from build123d import *

# Parameters (mm, degrees)
SKETCH_1_W           = 7.8
SKETCH_1_H           = 83.4
EXTRUDE_1_DEPTH      = 105
CUT_EXTRUDE_1_DEPTH  = 135.318278726
SKETCH_3_R           = 6
CUT_EXTRUDE_2_DEPTH  = 135.318278726
SKETCH_4_R           = 13.6
CUT_EXTRUDE_3_DEPTH  = 4
SKETCH_5_R           = 1.25
CUT_EXTRUDE_4_DEPTH  = 4
EXTRUDE_2_DEPTH      = 7.2
SKETCH_7_W           = 6
SKETCH_7_H           = 30
CUT_EXTRUDE_5_DEPTH  = 7.2
CUT_EXTRUDE_6_DEPTH  = 135.92798079
SKETCH_9_R           = 1.65
CUT_EXTRUDE_7_DEPTH  = 15
FILLET_1_R           = 5
CUT_EXTRUDE_8_DEPTH  = 135.92798079
CUT_EXTRUDE_10_DEPTH = 135.92798079
SKETCH_14_R          = 1.6
CUT_EXTRUDE_11_DEPTH = 135.92798079
SKETCH_15_R          = 3
CUT_EXTRUDE_12_DEPTH = 2


with BuildPart() as part:
    # 草图1 → 凸台-拉伸1 (new body)
    with BuildSketch(Plane(origin=(0, 0, 0), x_dir=(1, 0, 0), z_dir=(0, 1, 0))):
        with Locations((3.9, -41.7)):
            Rectangle(SKETCH_1_W, SKETCH_1_H)
    extrude(amount=EXTRUDE_1_DEPTH)

    # 草图2 → 切除-拉伸1 (cut, through all)
    with BuildSketch(Plane.ZY):
        with BuildLine():
            Line((0, 64.3), (0, 105))
            Line((0, 105), (32.622555426, 105))
            ThreePointArc((32.622555426, 105), (9.162180169, 90.380266115), (0, 64.3))
        make_face()
        with BuildLine():
            Line((83.4, 105), (83.4, 64.3))
            ThreePointArc((83.4, 64.3), (74.237819831, 90.380266115), (50.777444574, 105))
            Line((50.777444574, 105), (83.4, 105))
        make_face()
    extrude(amount=-CUT_EXTRUDE_1_DEPTH, mode=Mode.SUBTRACT)

    # 草图3 → 切除-拉伸2 (cut, through all)
    with BuildSketch(Plane.ZY):
        with Locations((41.7, 64.3)):
            Circle(SKETCH_3_R)
    extrude(amount=-CUT_EXTRUDE_2_DEPTH, mode=Mode.SUBTRACT)

    # 草图4 → 切除-拉伸3 (cut)
    with BuildSketch(Plane.ZY):
        with Locations((41.7, 64.3)):
            Circle(SKETCH_4_R)
    extrude(amount=-CUT_EXTRUDE_3_DEPTH, mode=Mode.SUBTRACT)

    # 草图5 → 切除-拉伸4 (cut)
    with BuildSketch(Plane.ZY.offset(-4)):
        with Locations((32.2, 64.3)):
            Circle(SKETCH_5_R)
        with Locations((51.2, 64.3)):
            Circle(SKETCH_5_R)
    extrude(amount=-CUT_EXTRUDE_4_DEPTH, mode=Mode.SUBTRACT)

    # 草图6 → 凸台-拉伸2 (add)
    with BuildSketch(Plane(origin=(7.8, 0, 0), x_dir=(0, 0, -1), z_dir=(1, 0, 0))):
        with BuildLine():
            ThreePointArc((-14.146415841, 30), (-26.974511893, 22.286540784), (-41.7, 19.6))
            Line((-41.7, 19.6), (-41.7, 0))
            Line((-41.7, 0), (0, 0))
            Line((0, 0), (0, 30))
            Line((0, 30), (-14.146415841, 30))
        make_face()
        with BuildLine():
            Line((-41.7, 0), (-41.7, 19.6))
            ThreePointArc((-41.7, 19.6), (-56.425488107, 22.286540784), (-69.253584159, 30))
            Line((-69.253584159, 30), (-83.4, 30))
            Line((-83.4, 30), (-83.4, 0))
            Line((-83.4, 0), (-41.7, 0))
        make_face()
    extrude(amount=EXTRUDE_2_DEPTH)

    # 草图7 → 切除-拉伸5 (cut)
    with BuildSketch(Plane(origin=(15, 0, 0), x_dir=(0, 0, -1), z_dir=(1, 0, 0))):
        with Locations((-80.4, 15)):
            Rectangle(SKETCH_7_W, SKETCH_7_H)
    extrude(amount=-CUT_EXTRUDE_5_DEPTH, mode=Mode.SUBTRACT)

    # 草图8 → 切除-拉伸6 (cut, through all)
    with BuildSketch(Plane.ZY):
        with BuildLine():
            Line((31.7, 17), (51.7, 17))
            ThreePointArc((51.7, 17), (55.235533906, 15.535533906), (56.7, 12))
            Line((56.7, 12), (56.7, 0))
            Line((56.7, 0), (26.7, 0))
            Line((26.7, 0), (26.7, 12))
            ThreePointArc((26.7, 12), (28.164466094, 15.535533906), (31.7, 17))
        make_face()
    extrude(amount=-CUT_EXTRUDE_6_DEPTH, mode=Mode.SUBTRACT)

    # 草图9 → 切除-拉伸7 (cut)
    with BuildSketch(Plane.XZ):
        with Locations(Location((7.5, 73.4, 0), (0, 0, 270))):
            Circle(SKETCH_9_R)
        with Locations(Location((7.5, 62.7, 0), (0, 0, 270))):
            Circle(SKETCH_9_R)
        with Locations(Location((7.5, 20.7, 0), (0, 0, 270))):
            Circle(SKETCH_9_R)
        with Locations(Location((7.5, 6, 0), (0, 0, 270))):
            Circle(SKETCH_9_R)
    extrude(amount=-CUT_EXTRUDE_7_DEPTH, mode=Mode.SUBTRACT)


with BuildPart() as body_2:
    # 镜向2: mirrored copy
    add(part.part.mirror(Plane(origin=(0, 0, 0), x_dir=(0, 0, 1), z_dir=(1, 0, 0))))

    # 圆角1
    fillet_1_edges = [body_2.edges().sort_by_distance(p)[0] for p in [
        (-11.4, 30, 14.146415841),
        (-11.4, 30, 69.253584159),
    ]]
    fillet(fillet_1_edges, radius=FILLET_1_R)

    # 草图10 → 切除-拉伸8 (cut, through all)
    with BuildSketch(Plane(origin=(0, 0, 0), x_dir=(0, 0, -1), z_dir=(1, 0, 0))):
        with BuildLine():
            ThreePointArc((-37.240706086, 94.065786869), (-59.594392776, 88.500786708), (-71.465786869, 68.759293914))
            ThreePointArc((-71.465786869, 68.759293914), (-68.859293916, 65.234213137), (-65.334213139, 67.840706089))
            ThreePointArc((-65.334213139, 67.840706089), (-55.908255092, 83.515569664), (-38.159293911, 87.934213139))
            ThreePointArc((-38.159293911, 87.934213139), (-34.634213133, 90.540706091), (-37.240706086, 94.065786869))
        make_face()
    extrude(amount=-CUT_EXTRUDE_8_DEPTH, mode=Mode.SUBTRACT)

    # 草图13 → 切除-拉伸10 (cut, through all)
    with BuildSketch(Plane(origin=(0, 0, 0), x_dir=(0, 0, -1), z_dir=(1, 0, 0))):
        with BuildLine():
            ThreePointArc((-56.294598294, 36.728714307), (-54.592965975, 31.672402134), (-51.772187936, 27.144151191))
            ThreePointArc((-51.772187936, 27.144151191), (-44.745463477, 26.353491098), (-43.954803385, 33.380215557))
            ThreePointArc((-43.954803385, 33.380215557), (-45.549156189, 35.939661742), (-46.51094837, 38.797577319))
            ThreePointArc((-46.51094837, 38.797577319), (-52.437204837, 42.654970775), (-56.294598294, 36.728714307))
        make_face()
    extrude(amount=-CUT_EXTRUDE_10_DEPTH, mode=Mode.SUBTRACT)

    # 草图14 → 切除-拉伸11 (cut, through all)
    with BuildSketch(Plane(origin=(0, 0, 0), x_dir=(0, 0, -1), z_dir=(1, 0, 0))):
        with Locations((-79.9, 7)):
            Circle(SKETCH_14_R)
        with Locations((-79.9, 22)):
            Circle(SKETCH_14_R)
    extrude(amount=-CUT_EXTRUDE_11_DEPTH, mode=Mode.SUBTRACT)

    # 草图15 → 切除-拉伸12 (cut)
    with BuildSketch(Plane(origin=(0, 0, 0), x_dir=(0, 0, -1), z_dir=(1, 0, 0))):
        with Locations((-79.9, 22)):
            Circle(SKETCH_15_R)
        with Locations((-79.9, 7)):
            Circle(SKETCH_15_R)
    extrude(amount=-CUT_EXTRUDE_12_DEPTH, mode=Mode.SUBTRACT)


solid = body_2.part
Check sheet for the modelled part. Datum: model origin and axes. Units: mm. A direction names the side the tool comes from. Give positions to 0.01 mm unless a question says otherwise; leave off trailing zeros. Loops run counter-clockwise (first coordinate to the right, second up) from the corner with the lowest first, then second, coordinate; pieces in that order, holes last. Notation, with made-up numbers: M -1.75,69.5 L 36.25,69.5 A8 ccw 36.25,81.5 Z; hole C 27,46.25 d2. An arc over 180 degrees is marked long. Use a Markdown table: item, result. Add a question column.
Q1. Sectioned sample at D-D, the plane z = 79.9. Record the cut outline in (x, y), then the cut area to 3 significant figures.
Q2. Go/stop test with flat-tipped pins: pin 1 (8 mm diameter, centred on x = -5, z = 67.5, fed in from +Y); pin 2 (3.5 mm diameter, centred on y = 7, z = 79.9, fed in from -X); pin 3 (4 mm diameter, centred on x = -7.5, z = 20.7, fed in from -Y); pin 4 (3 mm diameter, centred on y = 8, z = 80.5, fed in from +X). Record where each tip stops, or that it passes through.
Q3. Sectioned sample at C-C, the plane z = 62.7. Record the cut outline in (x, y).
Q4. Sectioned sample at B-B, the plane y = 91. Record the cut outline in (x, z).
Q5. Scan lines: line 1 along Z through (x, y) = (-7.5, 8.75); line 2 along Y through (x, z) = (-4.5, 79.9); line 3 along X through (y, z) = (10.25, 6). Record each from-to range of solid material in increasing order. Write a range as [from, to].
Q6. Tool access check on faces 1 (the cylindrical face through (-3.845, 31.74, 54.625)), 2 (the cylindrical face through (-11.45, 29.705, 69.389)), 3 (the cylindrical face through (-7.57, 7.4, 7.65)), 4 (the flat face through (-2, 5.7, 78.6)), 5 (the flat face through (-7, 6, 26.7)). Record the directions out of +Z, -Z, +X, -X, +Y, -Y that give a thin tool (end or side, any length) a straight path to the whole face; none if there is none.
Q7. Sectioned sample at A-A, the plane x = -12.25. Record the cut outline in (y, z).
Q8. Mould release check, pull along Y, two halves, no side actions. Record for faces 6 (the flat face through (-2, 20.7, 78.6)), 7 (the flat face through (-4, 32, 83.4)), 8 (the flat face through (-8, 15, 21)): pulls with the +Y half, pulls with the -Y half, needs draft (parallel to the pull), parting line crosses it, or undercut.
Verdict:
| question | item | result |
|---|---|---|
| 1 | outline | M -7.8,0 L 0,0 L 0,4 L -2,4 L -2,5.4 L -7.8,5.4 Z; M -7.8,8.6 L -2,8.6 L -2,10 L 0,10 L 0,19 L -2,19 L -2,20.4 L -7.8,20.4 Z; M -7.8,23.6 L -2,23.6 L -2,25 L 0,25 L 0,81.02 L -7.8,81.02 Z |
| 1 | area | 571 mm^2 |
| 2 | pin 1 | y = 99.85 |
| 2 | pin 2 | x = -7.8 |
| 2 | pin 3 | y = 0 |
| 2 | pin 4 | x = -2 |
| 3 | outline | M -15,0 L -9.15,0 L -9.15,15 L -5.85,15 L -5.85,0 L 0,0 L 0,75.71 L -7.8,75.71 L -7.8,25.27 L -15,25.27 Z; M -7.8,85.86 L 0,85.86 L 0,100.33 L -7.8,100.33 Z |
| 4 | outline | M -7.8,9.67 L 0,9.67 L 0,34.6 L -7.8,34.6 Z; M -7.8,55.59 L 0,55.59 L 0,73.73 L -7.8,73.73 Z |
| 5 | line 1 | [0, 4.35], [7.65, 19.05], [22.35, 26.7], [56.7, 61.05], [64.35, 71.75], [75.05, 83.4] |
| 5 | line 2 | [0, 5.4], [8.6, 20.4], [23.6, 81.02] |
| 5 | line 3 | [-15, -9.15], [-5.85, 0] |
| 6 | face 1 | +X, -X |
| 6 | face 2 | -X, +Y |
| 6 | face 3 | -Y |
| 6 | face 4 | +X |
| 6 | face 5 | +X, -X, -Y |
| 7 | outline | M 0,0 L 30,0 L 30,12.32 A5 ccw 28.89,15.47 A41.7 cw 28.89,67.93 A5 ccw 30,71.08 L 30,77.4 L 0,77.4 L 0,56.7 L 12,56.7 A5 cw 17,51.7 L 17,31.7 A5 cw 12,26.7 L 0,26.7 Z |
| 8 | face 6 | undercut |
| 8 | face 7 | needs draft |
| 8 | face 8 | pulls with the -Y half |
